```python
from build123d import *

# Parameters (mm, degrees)
F0_R     = 24
F0_R_2   = 13
F1_DEPTH = 2.2
F2_R     = 6
F3_DEPTH = 0.2
F4_COUNT = 20


with BuildPart() as f1:
    # F0 (on Top) → F1 (new body)
    with BuildSketch(Plane.XY):
        Circle(F0_R)
        Circle(F0_R_2, mode=Mode.SUBTRACT)
    extrude(amount=F1_DEPTH)


with BuildPart() as f3:
    # F2 (on Front) → F3 (new body, symmetric)
    with BuildSketch(Plane.XZ):
        with Locations((18.5, 6.2)):
            Circle(F2_R)
    extrude(amount=F3_DEPTH, both=True)


with BuildPart() as f4_1:
    # F4: instance of F3
    add(f3.part.rotate(Axis((0, 0, 3.1), (0, 0, 1)), 1 * 360 / F4_COUNT))


with BuildPart() as f4_2:
    # F4: instance of F3
    add(f3.part.rotate(Axis((0, 0, 3.1), (0, 0, 1)), 2 * 360 / F4_COUNT))


with BuildPart() as f4_3:
    # F4: instance of F3
    add(f3.part.rotate(Axis((0, 0, 3.1), (0, 0, 1)), 3 * 360 / F4_COUNT))


with BuildPart() as f4_4:
    # F4: instance of F3
    add(f3.part.rotate(Axis((0, 0, 3.1), (0, 0, 1)), 4 * 360 / F4_COUNT))


with BuildPart() as f4_5:
    # F4: instance of F3
    add(f3.part.rotate(Axis((0, 0, 3.1), (0, 0, 1)), 5 * 360 / F4_COUNT))


with BuildPart() as f4_6:
    # F4: instance of F3
    add(f3.part.rotate(Axis((0, 0, 3.1), (0, 0, 1)), 6 * 360 / F4_COUNT))


with BuildPart() as f4_7:
    # F4: instance of F3
    add(f3.part.rotate(Axis((0, 0, 3.1), (0, 0, 1)), 7 * 360 / F4_COUNT))


with BuildPart() as f4_8:
    # F4: instance of F3
    add(f3.part.rotate(Axis((0, 0, 3.1), (0, 0, 1)), 8 * 360 / F4_COUNT))


with BuildPart() as f4_9:
    # F4: instance of F3
    add(f3.part.rotate(Axis((0, 0, 3.1), (0, 0, 1)), 9 * 360 / F4_COUNT))


with BuildPart() as f4_10:
    # F4: instance of F3
    add(f3.part.rotate(Axis((0, 0, 3.1), (0, 0, 1)), 10 * 360 / F4_COUNT))


with BuildPart() as f4_11:
    # F4: instance of F3
    add(f3.part.rotate(Axis((0, 0, 3.1), (0, 0, 1)), 11 * 360 / F4_COUNT))


with BuildPart() as f4_12:
    # F4: instance of F3
    add(f3.part.rotate(Axis((0, 0, 3.1), (0, 0, 1)), 12 * 360 / F4_COUNT))


with BuildPart() as f4_13:
    # F4: instance of F3
    add(f3.part.rotate(Axis((0, 0, 3.1), (0, 0, 1)), 13 * 360 / F4_COUNT))


with BuildPart() as f4_14:
    # F4: instance of F3
    add(f3.part.rotate(Axis((0, 0, 3.1), (0, 0, 1)), 14 * 360 / F4_COUNT))


with BuildPart() as f4_15:
    # F4: instance of F3
    add(f3.part.rotate(Axis((0, 0, 3.1), (0, 0, 1)), 15 * 360 / F4_COUNT))


with BuildPart() as f4_16:
    # F4: instance of F3
    add(f3.part.rotate(Axis((0, 0, 3.1), (0, 0, 1)), 16 * 360 / F4_COUNT))


with BuildPart() as f4_17:
    # F4: instance of F3
    add(f3.part.rotate(Axis((0, 0, 3.1), (0, 0, 1)), 17 * 360 / F4_COUNT))


with BuildPart() as f4_18:
    # F4: instance of F3
    add(f3.part.rotate(Axis((0, 0, 3.1), (0, 0, 1)), 18 * 360 / F4_COUNT))


with BuildPart() as f4_19:
    # F4: instance of F3
    add(f3.part.rotate(Axis((0, 0, 3.1), (0, 0, 1)), 19 * 360 / F4_COUNT))


with BuildPart() as f1_1:
    add(f1.part)

    # F5: cut F3, F4_18, F4_16, F4_15, F4_17, F4_19, F4_13, F4_11, F4_8, F4_12, F4_14, F4_9, F4_10, F4_7, F4_5, F4_3, F4_4, F4_2, F4_1, F4_6
    add(f3.part, mode=Mode.SUBTRACT)
    add(f4_18.part, mode=Mode.SUBTRACT)
    add(f4_16.part, mode=Mode.SUBTRACT)
    add(f4_15.part, mode=Mode.SUBTRACT)
    add(f4_17.part, mode=Mode.SUBTRACT)
    add(f4_19.part, mode=Mode.SUBTRACT)
    add(f4_13.part, mode=Mode.SUBTRACT)
    add(f4_11.part, mode=Mode.SUBTRACT)
    add(f4_8.part, mode=Mode.SUBTRACT)
    add(f4_12.part, mode=Mode.SUBTRACT)
    add(f4_14.part, mode=Mode.SUBTRACT)
    add(f4_9.part, mode=Mode.SUBTRACT)
    add(f4_10.part, mode=Mode.SUBTRACT)
    add(f4_7.part, mode=Mode.SUBTRACT)
    add(f4_5.part, mode=Mode.SUBTRACT)
    add(f4_3.part, mode=Mode.SUBTRACT)
    add(f4_4.part, mode=Mode.SUBTRACT)
    add(f4_2.part, mode=Mode.SUBTRACT)
    add(f4_1.part, mode=Mode.SUBTRACT)
    add(f4_6.part, mode=Mode.SUBTRACT)


solid = f1_1.part
```
Input: part model. Units: mm. Frame: model coordinates. Give positions to 0.01 mm unless a question says otherwise; leave off trailing zeros.
1) Mould query, pull axis X, two halves, no side actions, for faces 1 (the cylindrical face through (-14.9, 10.8, 0.2)), 2 (the cylindrical face through (-23.977, 1.055, 1.085)). Classes: released by +X, released by -X, zero draft, split by the parting line, or undercut.
A:
face 1: undercut
face 2: split by the parting line
2) Contact query for flat-ended pins moving along their axis: pin 1 (1 mm diameter, centred on x = -16.5, z = 1, fed in from -Y); pin 2 (1 mm diameter, centred on x = -20.5, z = 1, fed in from +Y); pin 3 (1 mm diameter, centred on y = 10, z = 1, fed in from -X). Output: stop coordinate, or through.
A:
pin 1: stops at y = -17.89
pin 2: stops at y = 13.27
pin 3: stops at x = -22.04
3) Section query A-A on z = 1.7. Count the separate pieces of the cut face and the enclosed holes in it, and give its area (3 significant figures).
A:
separate pieces: 1
enclosed holes: 21
area: 1,220 mm2
4) Line query: L1, parallel to Y at x = -10, z = 1.8; L2, parallel to X at y = 17, z = 0.9; L3, parallel to Y at x = -13.5, z = 0.6. Output: solid intervals per line, ascending.
A:
L1: y = -21.82 to -14.1, -13.42 to -8.31, 8.31 to 13.42, 14.1 to 21.82
L2: x = -16.94 to -12.6, -12.1 to -5.73, -5.31 to -0.2, 0.2 to 5.31, 5.73 to 12.1, 12.6 to 16.94
L3: y = -19.84 to -10.06, -9.56 to 9.56, 10.06 to 19.84
